The model under review builds one solid part; all positions refer to its coordinate system, in mm. A direction names the side the tool comes from. Round coordinates to 2 decimals unless told otherwise and drop trailing zeros. Write each loop counter-clockwise with the first axis right and the second up, starting at its lowest first coordinate (ties: lowest second). Pieces come first, ordered by that corner, then holes. Notation, with made-up numbers: (59, 82.25) - (79, 82.25) arc R18 ccw to (79, 90.25) - close; hole circle Ø8 at (-3.75, 12). An arc over 180 degrees is marked (long way). Use one line per item in the form item = value.
from build123d import *

# Parameters (mm, degrees)
CHAMFER1_SIZE = 0.25


with BuildPart() as part:
    # Sketch4 → Revolve2 (revolve)
    with BuildSketch(Plane.XY):
        Polygon((2.5, 0), (8, 0), (8, 7.5), (6.366197724, 7.5), (6.366197724, 14.5), (8, 14.5), (8, 15.5), (2.5, 15.5), align=None)
    revolve(axis=Axis((0, 0, 0), (0, 1, 0)))

    # Chamfer1
    chamfer1_edges = [part.edges().sort_by_distance(p)[0] for p in [
        (-8, 15.5, 0),
        (-8, 14.5, 0),
        (-8, 7.5, 0),
        (-8, 0, 0),
    ]]
    chamfer(chamfer1_edges, length=CHAMFER1_SIZE)


solid = part.part
(1) Add section D-D on y = 5.75. Write out the cut boundary in (x, z), then the cut area to 3 significant figures.
Geometry results:
outline = circle Ø16 at (0, 0); hole circle Ø5 at (0, 0)
area = 181 mm2
(2) Add section B-B on x = 0. Write out the cut boundary in (y, z).
Geometry results:
outline = (0, -7.75) - (0.25, -8) - (7.25, -8) - (7.5, -7.75) - (7.5, -6.37) - (14.5, -6.37) - (14.5, -7.75) - (14.75, -8) - (15.25, -8) - (15.5, -7.75) - (15.5, -2.5) - (0, -2.5) - close; (0, 2.5) - (15.5, 2.5) - (15.5, 7.75) - (15.25, 8) - (14.75, 8) - (14.5, 7.75) - (14.5, 6.37) - (7.5, 6.37) - (7.5, 7.75) - (7.25, 8) - (0.25, 8) - (0, 7.75) - close
(3) Machinability: for faces 1 (the cylindrical face through (-0.54, 7.64, 2.44)), 2 (the flat face through (-6, 7.5, -3)), which of the approach directions +Z, -Z, +X, -X, +Y, -Y give a long, thin tool a straight path to every point of the face, cutting with its end or side? Answer none if there is none.
Geometry results:
face_1 = +Y, -Y
face_2 = none
(4) The part is to be moulded in two halves that separate along Y. For faces 3 (the cylindrical face through (-1.73, 3.8, 7.81)), 4 (the flat face through (2, 0, -2)), 5 (the cylindrical face through (-4.692, 11.049, -4.303)), say which applies: +Y half, -Y half, draft (parallel to the pull), parting line (faces both ways), or undercut.
Geometry results:
face_3 = draft
face_4 = -Y half
face_5 = undercut
(5) Insertion check: P1, Ø4, axis at x = -5, y = 4, coming from the -Z side; P2, Ø8, axis at y = 11, z = -2, coming from the +X side; P3, Ø4, axis at x = 6, y = 2, coming from the +Z side. Each pin has a flat end and moves straight along its axis. Give the tip position at first contact, or say it passes through.
Geometry results:
P1 = -7.42
P2 = 7.98
P3 = 6.93
(6) Add section C-C on y = 8.25. Write out the cut boundary in (x, z).
Geometry results:
outline = circle Ø12.73 at (0, 0); hole circle Ø5 at (0, 0)
(7) Add section A-A on z = 0. Write out the cut boundary in (x, y), then the cut area to 3 significant figures.
Geometry results:
outline = (-8, 0.25) - (-7.75, 0) - (-2.5, 0) - (-2.5, 15.5) - (-7.75, 15.5) - (-8, 15.25) - (-8, 14.75) - (-7.75, 14.5) - (-6.37, 14.5) - (-6.37, 7.5) - (-7.75, 7.5) - (-8, 7.25) - close; (2.5, 0) - (7.75, 0) - (8, 0.25) - (8, 7.25) - (7.75, 7.5) - (6.37, 7.5) - (6.37, 14.5) - (7.75, 14.5) - (8, 14.75) - (8, 15.25) - (7.75, 15.5) - (2.5, 15.5) - close
area = 147 mm2
(8) To check wall thickness, follow L1, parallel to Z at x = 0, y = 12; L2, parallel to Y at x = 2.75, z = -6.5. State the ranges of each line that lie inside material, in increasing order.
Geometry results:
L1 = -6.37 to -2.5, 2.5 to 6.37
L2 = 0 to 7.5, 14.5 to 15.5
